from build123d import *

# Parameters (mm, degrees)
F0_W        = 100
F0_H        = 136
F0_R        = 5
F0_R_2      = 3.75
F0_R_3      = 1.25
F0_W_2      = 12
F0_H_2      = 44
F1_DEPTH    = 15.5
F2_DEPTH    = 13
F4_R        = 3.75
F5_DEPTH    = 10
F6_T1_DEPTH = 211.4336597593
F6_T3_DEPTH = 311.4336597593
F7_SIZE     = 1.25
F8_SIZE     = 1.25
F9_W        = 12
F9_H        = 34
F9_W_2      = 20
F9_H_2      = 14
F10_DEPTH   = 13


# Not quite as in the source:
# - a fillet or chamfer that OpenCascade refuses, or shapes differently, is made with other operations: its cross-section is extruded or revolved along the edge and cut away or added


with BuildPart() as f1:
    # F0 (on Top) → F1 (new body)
    with BuildSketch(Plane.XY):
        Polygon((0, 196), (0, 0), (54, 0), (66, 0), (120, 0), (120, 196), align=None)
        with Locations((60, 108)):
            Rectangle(F0_W, F0_H, mode=Mode.SUBTRACT)
        with Locations((60, 186)):
            Circle(F0_R, mode=Mode.SUBTRACT)
        Polygon((54, 0), (0, 0), (0, 196), (120, 196), (120, 0), (66, 0), (66, -44), (140, -44), (140, 216), (-20, 216), (-20, -44), (54, -44), align=None)
        with Locations((-10, -34)):
            Circle(F0_R_2, mode=Mode.SUBTRACT)
        with Locations((130, -34)):
            Circle(F0_R_2, mode=Mode.SUBTRACT)
        with Locations((-10, 206)):
            Circle(F0_R_2, mode=Mode.SUBTRACT)
        with Locations((130, 206)):
            Circle(F0_R_2, mode=Mode.SUBTRACT)
        with Locations((130, -34)):
            Circle(F0_R_2)
        with Locations((130, -34)):
            Circle(F0_R_3, mode=Mode.SUBTRACT)
        with Locations((-10, -34)):
            Circle(F0_R_2)
        with Locations((-10, -34)):
            Circle(F0_R_3, mode=Mode.SUBTRACT)
        with Locations((-10, 206)):
            Circle(F0_R_2)
        with Locations((-10, 206)):
            Circle(F0_R_3, mode=Mode.SUBTRACT)
        with Locations((130, 206)):
            Circle(F0_R_2)
        with Locations((130, 206)):
            Circle(F0_R_3, mode=Mode.SUBTRACT)
        with Locations((60, -22)):
            Rectangle(F0_W_2, F0_H_2)
    extrude(amount=F1_DEPTH)

    # F0 (on Top) → F2 (cut)
    with BuildSketch(Plane.XY):
        Polygon((0, 196), (0, 0), (54, 0), (66, 0), (120, 0), (120, 196), align=None)
        with Locations((60, 108)):
            Rectangle(F0_W, F0_H, mode=Mode.SUBTRACT)
        with Locations((60, 186)):
            Circle(F0_R, mode=Mode.SUBTRACT)
    extrude(amount=F2_DEPTH, mode=Mode.SUBTRACT)

    # F4 (on offset) → F5 (cut)
    with BuildSketch(Plane.XY.offset(15.5)):
        with Locations((130, 208.356961264)):
            Circle(F4_R)
        with Locations((-10, 208.356961264)):
            Circle(F4_R)
        with Locations((130, -34)):
            Circle(F4_R)
        with Locations((-10, -34)):
            Circle(F4_R)
    extrude(amount=-F5_DEPTH, mode=Mode.SUBTRACT)

    # F6: chamfer of 10 on 4 edges, made by hand

    # F6_s2 → F6_t1 (cut)
    with BuildSketch(Plane.YZ.offset(-45.7168298797)):
        Polygon((216, 5.5), (206, 15.5), (216, 15.5), align=None)
        Polygon((-44, 5.5), (-34, 15.5), (-44, 15.5), align=None)
    extrude(amount=F6_T1_DEPTH, mode=Mode.SUBTRACT)

    # F6_s4 → F6_t3 (cut)
    with BuildSketch(Plane.XZ.offset(-241.7168298797)):
        Polygon((140, 5.5), (130, 15.5), (140, 15.5), align=None)
        Polygon((-10, 15.5), (-20, 5.5), (-20, 15.5), align=None)
    extrude(amount=F6_T3_DEPTH, mode=Mode.SUBTRACT)

    # F7
    f7_edges = [f1.edges().sort_by_distance(p)[0] for p in [
        (55, 186, 15.5),
    ]]
    chamfer(f7_edges, length=F7_SIZE)

    # F8
    f8_edges = [f1.edges().sort_by_distance(p)[0] for p in [
        (110, 108, 15.5),
        (60, 176, 15.5),
        (10, 108, 15.5),
        (60, 40, 15.5),
    ]]
    chamfer(f8_edges, length=F8_SIZE)

    # F9 (on face) → F10 (cut)
    with BuildSketch(Plane(origin=(0, 0, 0), x_dir=(1, 0, 0), z_dir=(0, 0, -1))):
        with Locations((60.329009831, 17)):
            Rectangle(F9_W, F9_H)
        with Locations((130, -163)):
            Rectangle(F9_W_2, F9_H_2)
    extrude(amount=-F10_DEPTH, mode=Mode.SUBTRACT)


solid = f1.part
Model file for the job. Use its own axes, mm. A direction names the side the tool comes from. Give positions to 0.01 mm unless a question says otherwise; leave off trailing zeros. Order: outer loops, then holes, each group sorted by start corner. A loop starts at its lowest first (then second) coordinate and runs counter-clockwise, first axis right, second up. Notation, with made-up numbers: (-17, 65.25) -> (16, 65.25) arc R11 ccw to (16, 70.25) -> close; hole circle Ø8 at (50.5, 57.25). An arc over 180 degrees is marked (long way). Use CSV: the item, a comma, the result in double quotes.
1. Drill centre lines: line 1 along Y through (x, z) = (130, 4.3); line 2 along X through (y, z) = (206, 4.1); line 3 along Y through (x, z) = (113.5, 4.5). Where is each one in solid material? Low to high. Write a range as from..to.
Outcome:
line 1,"-44..-35.25, -32.75..156, 170..204.75, 207.25..216"
line 2,"-20..-11.25, -8.75..128.75, 131.25..140"
line 3,"-44..0, 196..216"
2. Drop flat-ended pins along their axis: pin 1 (1.5 mm diameter, centred on x = 22.5, y = 175.5, fed in from -Z); pin 2 (1.5 mm diameter, centred on x = -10, y = 206, fed in from -Z); pin 3 (6 mm diameter, centred on x = -10, y = -34, fed in from +Z); pin 4 (1.4 mm diameter, centred on x = 69, z = 14, fed in from -Y). Give the stop position or say it passes through.
Outcome:
pin 1,"z = 13"
pin 2,"through"
pin 3,"z = 5.5"
pin 4,"y = -36.2"
3. Mould opens along Y. For faces 1 (the flat face through (6, 79, 13)), 2 (the flat face through (58.9, 211.1, 10.4)), 3 (the flat face through (58.9, -39.1, 10.4)), 4 (the cylindrical face through (127.236, -31.466, 9.459)) say: +Y half, -Y half, draft (parallel to the pull), parting line (faces both ways), or undercut.
Outcome:
face 1,"undercut"
face 2,"+Y half"
face 3,"-Y half"
face 4,"undercut"
4. Band-saw the part on C-C, the plane y = -15. Give the cut face in (x, z).
Outcome:
outline,"(-20, 0) -> (54.33, 0) -> (54.33, 13) -> (66.33, 13) -> (66.33, 0) -> (140, 0) -> (140, 5.5) -> (130, 15.5) -> (-10, 15.5) -> (-20, 5.5) -> close"
5. Band-saw the part on A-A, the plane y = 186. Give the cut face in (x, z).
Outcome:
outline,"(-20, 0) -> (0, 0) -> (0, 13) -> (55, 13) -> (55, 14.25) -> (53.75, 15.5) -> (-10, 15.5) -> (-20, 5.5) -> close; (65, 13) -> (120, 13) -> (120, 0) -> (140, 0) -> (140, 5.5) -> (130, 15.5) -> (66.25, 15.5) -> (65, 14.25) -> close"
6. Band-saw the part on D-D, the plane z = 8. Give the cut face in (x, y).
Outcome:
outline,"(-17.5, -41.5) -> (137.5, -41.5) -> (137.5, 156) -> (120, 156) -> (120, 0) -> (66.33, 0) -> (66.33, -34) -> (54.33, -34) -> (54.33, 0) -> (0, 0) -> (0, 196) -> (120, 196) -> (120, 170) -> (137.5, 170) -> (137.5, 213.5) -> (-17.5, 213.5) -> close; hole circle Ø7.5 at (-10, -34); hole circle Ø7.5 at (-10, 208.36); hole circle Ø7.5 at (130, -34); hole circle Ø7.5 at (130, 208.36)"
7. Band-saw the part on B-B, the plane x = 60. Give the cut face in (y, z), then the cut area to 3 significant figures.
Outcome:
outline,"(-44, 0) -> (-34, 0) -> (-34, 13) -> (40, 13) -> (40, 14.25) -> (38.75, 15.5) -> (-34, 15.5) -> (-44, 5.5) -> close; (176, 13) -> (181, 13) -> (181, 14.25) -> (179.75, 15.5) -> (177.25, 15.5) -> (176, 14.25) -> close; (191, 13) -> (196, 13) -> (196, 0) -> (216, 0) -> (216, 5.5) -> (206, 15.5) -> (192.25, 15.5) -> (191, 14.25) -> close"
area,"572 mm²"
8. 3-axis set-ups, long thin cutter, end or side, ignore diameter. For faces 5 (the flat face through (130, 170, 6)), 6 (the cylindrical face through (129.187, 204.696, 9.459)), 7 (the flat face through (59, 34, 15.5)), 8 (the flat face through (54.329, -17, 6)): which of +Z, -Z, +X, -X, +Y, -Y reach the whole face in a straight line?
Outcome:
face 5,"-Z, +X"
face 6,"+Z"
face 7,"+Z, +X, -X, +Y, -Y"
face 8,"-Z"
